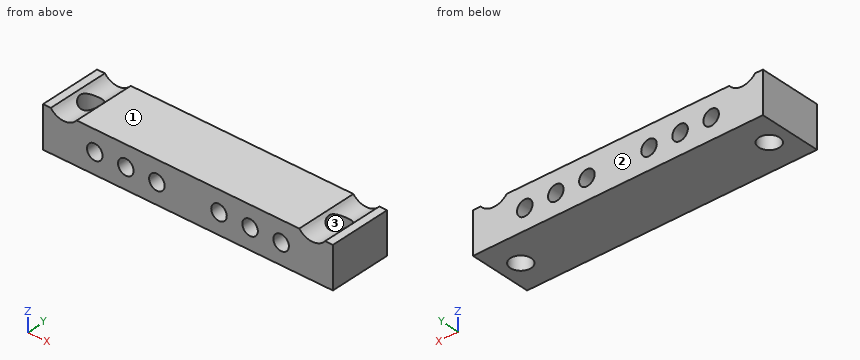
from build123d import *

# Parameters (mm, degrees)
CROQUIS1_W              = 28
CROQUIS1_H              = 6
CROQUIS1_R              = 1
SALIENTE_EXTRUIR1_DEPTH = 4
CROQUIS2_R              = 1.6
CROQUIS2_R_2            = 0.75
CORTAR_EXTRUIR1_DEPTH   = 6


with BuildPart() as part:
    # Croquis1 → Saliente-Extruir1 (new body)
    with BuildSketch(Plane.XY):
        with Locations((14, 3)):
            Rectangle(CROQUIS1_W, CROQUIS1_H)
        with Locations((2, 3)):
            Circle(CROQUIS1_R, mode=Mode.SUBTRACT)
        with Locations(Location((26, 3, 0), (0, 0, 180))):
            Circle(CROQUIS1_R, mode=Mode.SUBTRACT)
    extrude(amount=SALIENTE_EXTRUIR1_DEPTH)

    # Croquis2 → Cortar-Extruir1 (cut)
    with BuildSketch(Plane.XZ):
        with Locations((2, 5)):
            Circle(CROQUIS2_R)
        with Locations(Location((11, 2, 0), (0, 0, 270))):
            Circle(CROQUIS2_R_2)
        with Locations(Location((8, 2, 0), (0, 0, 270))):
            Circle(CROQUIS2_R_2)
        with Locations(Location((5, 2, 0), (0, 0, 270))):
            Circle(CROQUIS2_R_2)
        with Locations(Location((23, 2, 0), (0, 0, 90))):
            Circle(CROQUIS2_R_2)
        with Locations(Location((20, 2, 0), (0, 0, 90))):
            Circle(CROQUIS2_R_2)
        with Locations(Location((17, 2, 0), (0, 0, 90))):
            Circle(CROQUIS2_R_2)
        with Locations((26, 5)):
            Circle(CROQUIS2_R)
    extrude(amount=-CORTAR_EXTRUIR1_DEPTH, mode=Mode.SUBTRACT)


solid = part.part
Source: CAD feature listing. Evaluate the final solid. Frame: model axes, mm. Face numbers are marked on the shaded views. Coordinates: 2 decimals unless noted, no trailing zeros. Loops run counter-clockwise (first coordinate to the right, second up) from the corner with the lowest first, then second, coordinate; pieces in that order, holes last. Notation, with made-up numbers: (-26.5, 50.25) - (-15.5, 50.25) arc R17 ccw to (-15.5, 54.25) - close; hole circle Ø7 at (20.25, 26.5). An arc over 180 degrees is marked (long way). One line per item, written item: value. Start each with the question number.
1. Section D-D (y = 5.5). Return the cut outline in (x, z).
2. Mould query, pull axis Y, two halves, no side actions, for the marked faces 1, 2 and 3. Classes: pulls with the +Y half, pulls with the -Y half, needs draft (parallel to the pull), parting line crosses it, or undercut.
3. Section C-C (x = 26). Return the cut outline in (y, z).
4. Contact query for a flat-ended pin moving along its axis: P1, Ø1.2, axis at x = 17, z = 2, coming from the +Y side. Output: stop coordinate, or through.
5. Section A-A (z = 2). State how many separate pieces and enclosed holes the cut face has, and give its area (3 significant figures).
6. Ray query, L1, parallel to Y at x = 26, z = 1; L2, parallel to X at y = 3.75, z = 0.7; L3, parallel to Z at x = 4.5, y = 2.5. Return the intervals inside material, ascending.
Verdict:
1. outline: (0, 0) - (28, 0) - (28, 4) - (27.25, 4) arc R1.6 cw to (24.75, 4) - (3.25, 4) arc R1.6 cw to (0.75, 4) - (0, 4) - close; hole circle Ø1.5 at (5, 2); hole circle Ø1.5 at (8, 2); hole circle Ø1.5 at (11, 2); hole circle Ø1.5 at (17, 2); hole circle Ø1.5 at (20, 2); hole circle Ø1.5 at (23, 2)
2. face 1: needs draft
2. face 2: pulls with the +Y half
2. face 3: undercut
3. outline: (0, 0) - (2, 0) - (2, 3.4) - (0, 3.4) - close; (4, 0) - (6, 0) - (6, 3.4) - (4, 3.4) - close
4. P1: passes through
5. separate pieces: 7
5. enclosed holes: 2
5. area: 108 mm2
6. L1: y = 0 to 2, 4 to 6
6. L2: x = 0 to 1.34, 2.66 to 25.34, 26.66 to 28
6. L3: z = 0 to 1.44, 2.56 to 4
